from build123d import *


with BuildPart() as f1:
    # F0 (on Top) → F1 (revolve)
    with BuildSketch(Plane.XY):
        Polygon((68.077475, 22.601893), (68.077475, 15.875), (187.976122, 15.875), (187.976122, 20.58054), (187.457475, 20.061893), (184.917475, 22.601893), (179.837475, 22.601893), (177.297475, 20.061893), (174.757475, 22.601893), (169.677475, 22.601893), (167.137475, 20.061893), (164.597475, 22.601893), (159.517475, 22.601893), (156.977475, 20.061893), (154.437475, 22.601893), (149.357475, 22.601893), (146.817475, 20.061893), (144.277475, 22.601893), (139.197475, 22.601893), (136.657475, 20.061893), (134.117475, 22.601893), (129.037475, 22.601893), (126.497475, 20.061893), (123.957475, 22.601893), (118.877475, 22.601893), (116.337475, 20.061893), (113.797475, 22.601893), (108.717475, 22.601893), (106.177475, 20.061893), (103.637475, 22.601893), (98.557475, 22.601893), (96.017475, 20.061893), (93.477475, 22.601893), (88.397475, 22.601893), (85.857475, 20.061893), (83.317475, 22.601893), (78.237475, 22.601893), (75.697475, 20.061893), (73.157475, 22.601893), align=None)
        with BuildLine():
            Line((187.976122, 20.58054), (187.976122, 15.875))
            Line((187.976122, 15.875), (254, 15.875))
            Line((254, 15.875), (254, 18.475244))
            ThreePointArc((254, 18.475244), (251.94463, 20.004972), (249.747694, 21.323336))
            ThreePointArc((249.747694, 21.323336), (236.586927, 18.688808), (223.179117, 19.302912))
            Line((223.179117, 19.302912), (203.661054, 22.601893))
            Line((203.661054, 22.601893), (202.15936, 21.992272))
            Line((202.15936, 21.992272), (189.997475, 22.601893))
            Line((189.997475, 22.601893), (187.976122, 20.58054))
        make_face()
        with BuildLine():
            Line((254, 15.875), (254, 0))
            Line((254, 0), (263.476824, 0))
            Line((263.476824, 0), (263.082504, 2.533392))
            ThreePointArc((263.082504, 2.533392), (260.005937, 11.338789), (254, 18.475244))
            Line((254, 18.475244), (254, 15.875))
        make_face()
    revolve(axis=Axis((127, 0, 0), (1, 0, 0)))


solid = f1.part
Could you check a few things on this model? Use its own coordinates, in mm. A direction names the side the tool comes from. Give positions to 0.01 mm unless a question says otherwise; leave off trailing zeros. Use CSV: the item, a comma, the result in double quotes. Start each with the question number.
Item 1: If we mould it in two halves opening along X, with no side actions, what happens to faces 1 (the face through (254, 0, 0)), 2 (the face through (162.022, -16.659, 15.275)), 3 (the face through (126.621, -4.376, -19.705))? For each: pulls with the +X half, pulls with the -X half, needs draft (parallel to the pull), parting line crosses it, or undercut.
Item 2: If I drill on line 1 along Z through (x, y) = (113.5, 0) (3 decimals); line 2 along Y through (x, z) = (143, -1.5); line 3 along Z through (x, y) = (80, -4), over which ranges is the centre line in solid material (lowest first)?
Item 3: For faces 4 (the face through (187.581, -4.376, -19.705)), 5 (the face through (182.342, -16.659, 15.275)), which set-ups out of +Z, -Z, +X, -X, +Y, -Y let a thin tool reach every point of the face, with its end or its side?
Item 4: I'm going to push flat-ended pins straight in: pin 1 (12 mm diameter, centred on x = 220, y = -14.5, fed in from -Z); pin 2 (6 mm diameter, centred on x = 200.5, y = -18, fed in from -Z); pin 3 (10 mm diameter, centred on x = 143, y = 3.5, fed in from +Z). Where does each tip first touch, or does it pass through?
Findings:
1,face 1,"pulls with the -X half"
1,face 2,"needs draft"
1,face 3,"undercut"
2,line 1,"z = -22.602 to -15.875, 15.875 to 22.602"
2,line 2,"y = -22.55 to -15.8, 15.8 to 22.55"
2,line 3,"z = -22.25 to -15.36, 15.36 to 22.25"
3,face 4,"none"
3,face 5,"+X, -X"
4,pin 1,"stops at z = -18.14"
4,pin 2,"stops at z = -16.2"
4,pin 3,"stops at z = 22.6"
